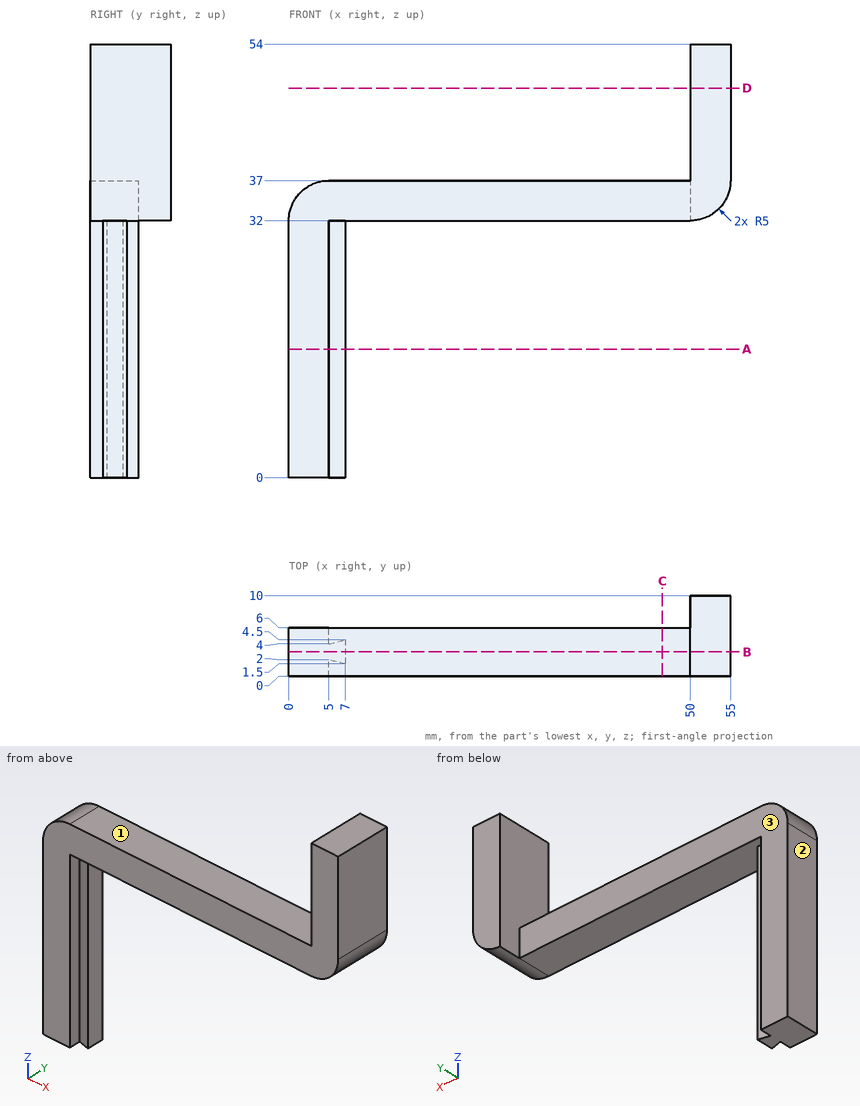
Print and shaded views of the part. All mm, measured from the part's lowest x, y and z. A direction names the side the tool comes from. Round coordinates to 2 decimals unless told otherwise and drop trailing zeros. Order: outer loops, then holes, each group sorted by start corner. A loop starts at its lowest first (then second) coordinate and runs counter-clockwise, first axis right, second up. Notation, with made-up numbers: (48.5, 82) - (99.5, 82) arc R23 cw to (99.5, 97) - close; hole circle Ø4 at (61, 0.5). An arc over 180 degrees is marked (long way). Use a Markdown table: item, result.
1) Flat gauge pins, fed straight in: pin 1 Ø1 at (y, z) = (4.5, 12.5) entering from +X; pin 2 Ø2 at (x, y) = (27, 6.5) entering from +Z; pin 3 Ø3 at (y, z) = (6, 45.5) entering from -X; pin 4 Ø1 at (y, z) = (6, 10.5) entering from -X. Where does each tip first touch, or does it go through?
Recorded:
| item | result |
|---|---|
| pin 1 | stops at x = 7 |
| pin 2 | stops at z = 37 |
| pin 3 | stops at x = 50 |
| pin 4 | stops at x = 0 |
2) Saw through at B-B on y = 3. Write the cut outline in (x, z).
Recorded:
| item | result |
|---|---|
| outline | (0, 0) - (7, 0) - (7, 32) - (50, 32) arc R5 ccw to (55, 37) - (55, 54) - (50, 54) - (50, 37) - (5, 37) arc R5 ccw to (0, 32) - close |
3) Wall check: L1, parallel to Y at x = 22, z = 36; L2, parallel to X at y = 4, z = 45; L3, parallel to Z at x = 37, y = 5.5. Give the ranges that are in metal, low to high.
Recorded:
| item | result |
|---|---|
| L1 | y = 0 to 6 |
| L2 | x = 50 to 55 |
| L3 | z = 32 to 37 |
4) Saw through at A-A on z = 16. Write the cut outline in (x, y).
Recorded:
| item | result |
|---|---|
| outline | (0, 0) - (5, 0) - (5, 2) - (7, 1.5) - (7, 4.5) - (5, 4) - (5, 6) - (0, 6) - close |
5) Saw through at D-D on z = 48.5. Write the cut outline in (x, y).
Recorded:
| item | result |
|---|---|
| outline | (50, 0) - (55, 0) - (55, 10) - (50, 10) - close |
6) Tool access for the marked faces 1, 2 and 3: list every direction of +Z, -Z, +X, -X, +Y, -Y with a clear straight run to the whole face (end or side of a thin tool).
Recorded:
| item | result |
|---|---|
| face 1 | +Z, -X, +Y, -Y |
| face 2 | +Z, -Z, -X, +Y, -Y |
| face 3 | +Z, -Z, -X, +Y |
7) Saw through at C-C on x = 46.5. Write the cut outline in (y, z).
Recorded:
| item | result |
|---|---|
| outline | (0, 32) - (6, 32) - (6, 37) - (0, 37) - close |
